Autodesk Inventor part; units mm, degrees
ref_plane "YZ Plane" through (0, 0, 0) normal (1, 0, 0) x (0, 1, 0)
ref_plane "XZ Plane" through (0, 0, 0) normal (0, 1, 0) x (-1, 0, 0)
ref_plane "XY Plane" through (0, 0, 0) normal (0, 0, 1) x (1, 0, 0)
ref_plane "Work Plane1" through (-82.8143, 19.6092, -42.8892) normal (0, 1, 0) x (0.9999998, 0, -0.0005571)
sketch "Sketch1" plane through (-82.8143, 19.6092, -42.8892) normal (0, 1, 0) x (0.9999998, 0, -0.0005571)
  arc A0 (1.5, -2) -> (-1.5, -2) centre (0, 0) ccw
  line L0 (-1.5, -2) -> (-1.1358, -2)
  line L1 (-1.1358, -2) -> (1.1358, -2)
  line L2 (1.1358, -2) -> (1.5, -2)
  line L3 (1.1358, -2.2) -> (-1.1358, -2.2)
  line L4 (-1.1358, -2.2) -> (-1.5652, -2.2)
  arc A1 (1.5652, -2.2) -> (-1.5652, -2.2) centre (0, 0) ccw
  line L5 (1.5652, -2.2) -> (1.1358, -2.2)
  circle A2 centre (0, 0) radius 12.5
  point P0 (82.7904, -42.9353)
  dimension "d0" = 0.2
  dimension "d1" = 25
extrude "Extrusion1" add sketch "Sketch1" against normal blind 13 contours A2
sketch "Sketch2" plane through (-81.2478, 6.6092, -40.69) normal (-0.0005571, 0, -0.9999998) x (-0.9999998, 0, 0.0005571)
  spline S0 degree 2 poles (3.0652, 12.8) (2.8756, 12.9138) (2.701, 13) knots 0 0 0 1 1 1 weights 1.078346 1.041437 1
  line L0 (3.0652, -2) -> (3.0652, 12.8)
  arc A0 (0.0652, -2) -> (3.0652, -2) centre (1.5652, 0.5981) ccw
  line L1 (0.0652, 12.8) -> (0.0652, -2)
  spline S1 degree 2 poles (0.4295, 13) (0.2549, 12.9138) (0.0652, 12.8) knots 0 0 0 1 1 1 weights 1 1.041437 1.078346
  line L2 (2.701, 13) -> (0.4295, 13)
  circle A1 centre (1.5652, 10) radius 1.5
  circle A2 centre (1.5652, 3) radius 1.5
  line L3 (-10.9348, 0) -> (14.0652, 0)
  point P0 (-81.2252, -6.6092)
  dimension "d4" = 3
  dimension "d5" = 3
  dimension "d6" = 3
  dimension "d7" = 3
extrude "Extrusion2" cut sketch "Sketch2" against normal blind 13 contours A1 | A2
sketch "Sketch3" plane through (-82.8143, 19.6092, -42.8892) normal (0, 1, 0) x (1, 0, 0)
  circle A0 centre (0, 0) radius 12.5
  line L0 (1.5665, -2.1991) -> (-1.564, -2.2009)
  arc A1 (1.5665, -2.1991) -> (-1.564, -2.2009) centre (0, 0) ccw
  point P0 (82.8143, -42.8892)
extrude "Extrusion3" add sketch "Sketch3" along normal blind 3 contours A0 | L0 A1
move faces "Move1" translate (0, 15, 0) faces at (-80.4474, 22.6092, -41.4544)
sketch "Sketch5" plane through (-82.8143, 37.6092, -42.8892) normal (0, 1, 0) x (1, 0, 0)
  line L0 (6, 6) -> (-6, 6)
  line L1 (-6, 6) -> (-6, -6)
  line L2 (-6, -6) -> (6, -6)
  line L3 (6, -6) -> (6, 6)
  line L4 (6, 6) -> (-6, -6) construction
  line L5 (-6, 6) -> (6, -6) construction
  point P0 (82.8143, -42.8892)
  point P1 (0, 0)
  dimension "d18" = 12
  dimension "d19" = 12
extrude "Extrusion5" cut sketch "Sketch5" against normal blind 20
fillet "Fillet2" radius 1 4 edges at (-82.8143, 37.6092, -36.8892) (-76.8143, 37.6092, -42.8892) (-82.8143, 37.6092, -48.8892) (-88.8143, 37.6092, -42.8892)
sketch "Sketch6" plane through (-82.8143, 17.6092, -42.8892) normal (0, 1, 0) x (1, 0, 0)
  line L0 (-1.1168, -2.2006) -> (-1.1147, -6)
  line L1 (-1.564, -2.2009) -> (-1.1168, -2.2006)
  arc A0 (1.5665, -2.1991) -> (-1.564, -2.2009) centre (0, 0) ccw
  line L2 (1.1193, -2.1994) -> (1.5665, -2.1991)
  line L3 (1.1214, -6) -> (1.1193, -2.1994)
  line L4 (6, -6) -> (1.1214, -6)
  line L5 (6, 6) -> (6, -6)
  line L6 (-6, 6) -> (6, 6)
  line L7 (-6, -6) -> (-6, 6)
  line L8 (-1.1147, -6) -> (-6, -6)
  line L9 (6, -6) -> (-6, -6)
ref_plane "Work Plane2" through (4.3942, -24.185, 88.7409) normal (0, 1, 0) x (0.9994696, 0, 0.0325661)
sketch "Sketch7" plane through (4.3942, -24.185, 88.7409) normal (0, 1, 0) x (0.9994696, 0, 0.0325661)
  point P0 (-7.2818, 88.5508)
equation "\"d7\" = d6"
properties part number "Motor-Driver Coupler"
Could you check a few things on this model? Use its own coordinates, in mm. A direction names the side the tool comes from. Round coordinates to 2 decimals unless told otherwise and drop trailing zeros. Loops run counter-clockwise (first coordinate to the right, second up) from the corner with the lowest first, then second, coordinate; pieces in that order, holes last. Notation, with made-up numbers: M 18.25,30 L 60.25,30 A17 cw 60.25,60 Z; hole C 85,67.5 d8. An arc over 180 degrees is marked long. Write item = value, one per line.
1. Thinking about a two-plate mould opening in Z: for faces 1 (the face through (-70.89, 21.89, -39.14)), 2 (the face through (-82.72, 12.186, -45.588)), 3 (the face through (-83, 17.609, -46)), which applies, +Z half, -Z half, draft (parallel to the pull), parting line (faces both ways), or undercut?
Results below:
face_1 = parting line
face_2 = undercut
face_3 = undercut
2. Which directions (+Z, -Z, +X, -X, +Y, -Y) give clear straight access to the entire face, cutting with the end or side of a thin tool? Please do faces 4 (the face through (-83, 6.609, -40)), 5 (the face through (-83, 27, -48.889)).
Results below:
face_4 = +Z, -Z, +X, -X, -Y
face_5 = +Y
3. I want a section at A-A, the plane x = -80.5. Write out the boundary of the cut face in (y, z).
Results below:
outline = M 6.61,-55.17 L 37.61,-55.17 L 37.61,-49.89 A1 ccw 36.61,-48.89 L 17.61,-48.89 L 17.61,-44.28 L 6.61,-44.28 Z; M 6.61,-41.5 L 17.61,-41.5 L 17.61,-36.89 L 36.61,-36.89 A1 ccw 37.61,-35.89 L 37.61,-30.61 L 6.61,-30.61 Z
4. I want a section at B-B, the plane y = 9. Write out the boundary of the cut face in (x, z), and give its area (3 significant figures).
Results below:
outline = M -84.38,-40.69 L -84.18,-40.69 L -84.18,-30.46 A12.5 ccw long -81.44,-30.47 L -81.44,-40.69 L -81.25,-40.69 A2.7 cw long Z
area = 441 mm²
5. I need wall thicknesses on probe 1 along X at (y, z) = (16.5, -43); probe 2 along Y at (x, z) = (-77.75, -39.5); probe 3 along Z at (x, y) = (-83.25, 20). Which ranges of each line are inside material? Lowest first, please.
Results below:
probe_1 = -95.31 to -85.51, -80.12 to -70.31
probe_2 = 6.61 to 17.61
probe_3 = -55.38 to -48.89, -36.89 to -30.4
6. Will these pins go through, and if not, where does the flat tip stop? P1, Ø3.5, axis at x = -80.5, y = 31, coming from the +Z side; P2, Ø6, axis at x = -73, y = 20.5, coming from the +Z side; P3, Ø6, axis at y = 24.5, z = -50, coming from the -X side.
Results below:
P1 = -30.4
P2 = -32.41
P3 = -94.62
7. I want a section at D-D, the plane x = -87. Write out the boundary of the cut face in (y, z).
Results below:
outline = M 6.61,-54.67 L 37.61,-54.67 L 37.61,-49.89 A1 ccw 36.61,-48.89 L 17.61,-48.89 L 17.61,-36.89 L 36.61,-36.89 A1 ccw 37.61,-35.89 L 37.61,-31.11 L 6.61,-31.11 Z
8. I want a section at C-C, the plane y = 32. Write out the boundary of the cut face in (x, z), and give its area (3 significant figures).
Results below:
outline = C -82.81,-42.89 d25; hole M -88.81,-48.89 L -76.81,-48.89 L -76.81,-36.89 L -88.81,-36.89 Z
area = 347 mm²
